Answer from the drawing. Dimensions are ordinates in mm from the lowest x, y and z of the part. A direction names the side the tool comes from. Coordinates: 2 decimals unless noted, no trailing zeros. Loops run counter-clockwise (first coordinate to the right, second up) from the corner with the lowest first, then second, coordinate; pieces in that order, holes last. Notation, with made-up numbers: (-33, -36.5) -> (-18, -36.5) arc R27 ccw to (-18, -13.5) -> close; hole circle Ø3 at (64, 15.5). An arc over 180 degrees is marked (long way). Use a Markdown table: item, result.
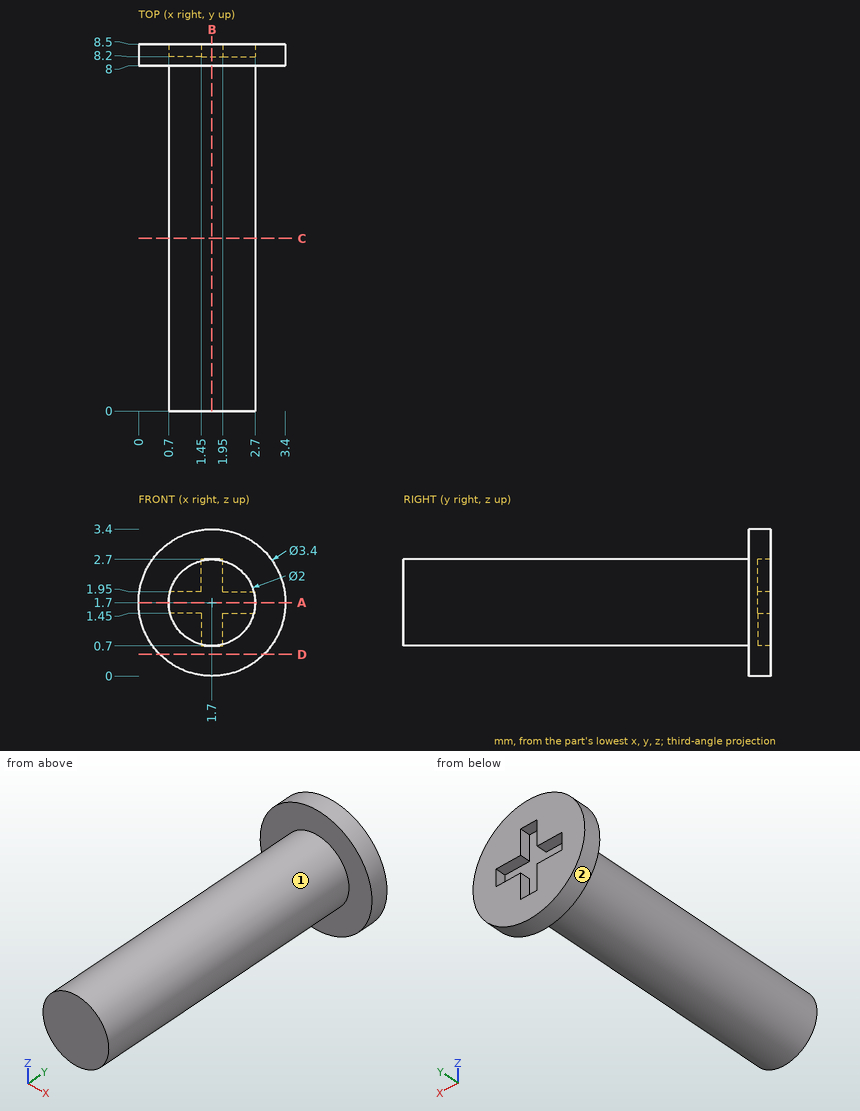
Q1. Section A-A on z = 1.7 is taken. Determine the outline of the cut face in (x, y).
Solved:
| item | result |
|---|---|
| outline | (0, 8) -> (0.7, 8) -> (0.7, 0) -> (2.7, 0) -> (2.7, 8) -> (3.4, 8) -> (3.4, 8.5) -> (2.7, 8.5) -> (2.7, 8.2) -> (0.7, 8.2) -> (0.7, 8.5) -> (0, 8.5) -> close |
Q2. For the marked faces 1 and 2, determine the directions among +Z, -Z, +X, -X, +Y, -Y from which every point of the face is accessible in a straight line to the end or side of a thin tool.
Solved:
| item | result |
|---|---|
| face 1 | -Y |
| face 2 | +Y, -Y |
Q3. Consider line 1 (Y direction, x = 0.6, z = 0.7); line 2 (Y direction, x = 1.5, z = 1.6); line 3 (X direction, y = 8.25, z = 2.3). Determine where each line is inside the solid, lowest interval first. Write a range as [from, to].
Solved:
| item | result |
|---|---|
| line 1 | [8, 8.5] |
| line 2 | [0, 8.2] |
| line 3 | [0.11, 1.45], [1.95, 3.29] |
Q4. Section B-B on x = 1.7 is taken. Determine the outline of the cut face in (y, z), and give its area (3 significant figures).
Solved:
| item | result |
|---|---|
| outline | (0, 0.7) -> (8, 0.7) -> (8, 0) -> (8.5, 0) -> (8.5, 0.7) -> (8.2, 0.7) -> (8.2, 2.7) -> (8.5, 2.7) -> (8.5, 3.4) -> (8, 3.4) -> (8, 2.7) -> (0, 2.7) -> close |
| area | 17.1 mm² |
Q5. Section D-D on z = 0.5 is taken. Determine the outline of the cut face in (x, y), and give its area (3 significant figures).
Solved:
| item | result |
|---|---|
| outline | (0.5, 8) -> (2.9, 8) -> (2.9, 8.5) -> (0.5, 8.5) -> close |
| area | 1.20 mm² |
Q6. Section C-C on y = 4 is taken. Determine the outline of the cut face in (x, z).
Solved:
| item | result |
|---|---|
| outline | circle Ø2 at (1.7, 1.7) |
Q7. Given pin 1 Ø2 at (x, y) = (1.5, 3.5) entering from -Z, flat-ended and moving along its own axis, determine where the tip first touches the part or whether it passes through.
Solved:
| item | result |
|---|---|
| pin 1 | z = 0.7 |
